For this review, use the dimensioned drawing (mm, ordinates from the lowest corner) and the shaded views. A direction names the side the tool comes from. Give positions to 0.01 mm unless a question says otherwise; leave off trailing zeros. Order: outer loops, then holes, each group sorted by start corner. A loop starts at its lowest first (then second) coordinate and runs counter-clockwise, first axis right, second up. Notation, with made-up numbers: (-24.5, 76.5) - (10.5, 76.5) arc R22 cw to (10.5, 87.5) - close; hole circle Ø5 at (26.25, -16.75). An arc over 180 degrees is marked (long way). One line per item, written item: value.
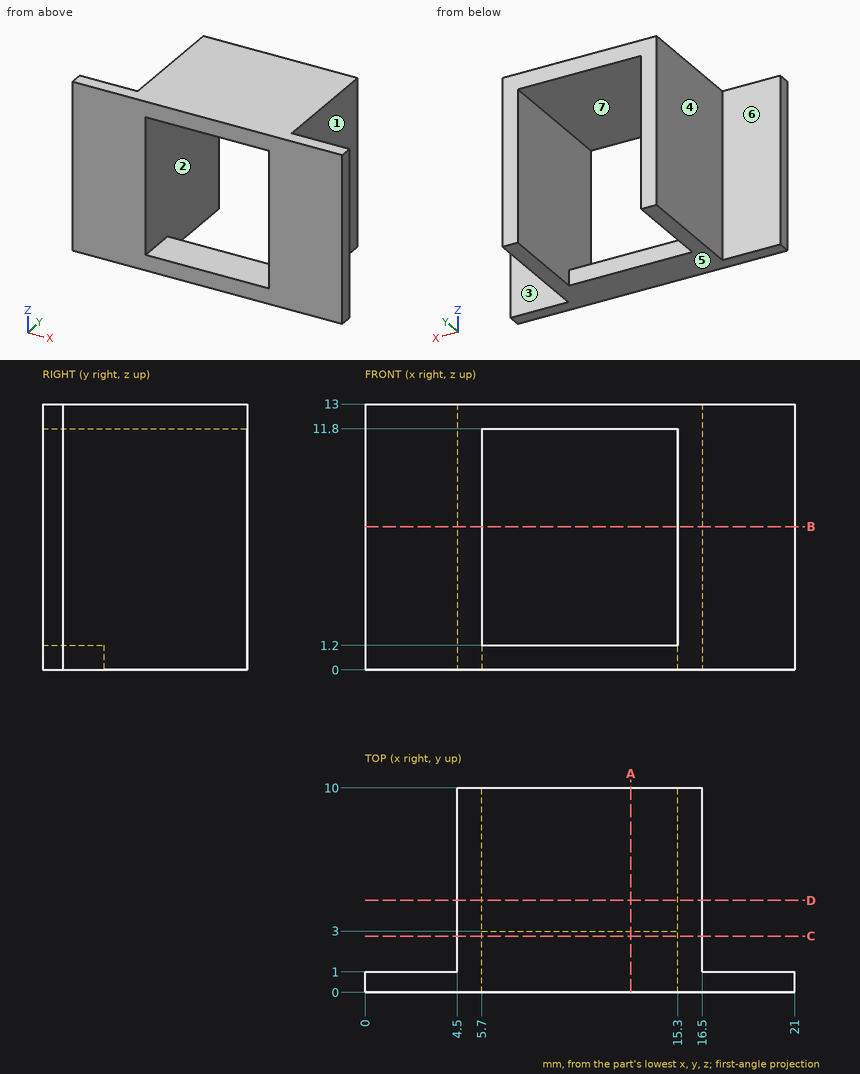
(1) Take a section at D-D (y = 4.5). Write out the cut boundary in (x, z).
Answers below:
outline: (4.5, 0) - (5.7, 0) - (5.7, 11.8) - (15.3, 11.8) - (15.3, 0) - (16.5, 0) - (16.5, 13) - (4.5, 13) - close
(2) Take a section at C-C (y = 2.75). Write out the cut boundary in (x, z).
Answers below:
outline: (4.5, 0) - (16.5, 0) - (16.5, 13) - (4.5, 13) - close; hole (5.7, 1.2) - (15.3, 1.2) - (15.3, 11.8) - (5.7, 11.8) - close
(3) Take a section at B-B (z = 7). Write out the cut boundary in (x, y).
Answers below:
outline: (0, 0) - (5.7, 0) - (5.7, 10) - (4.5, 10) - (4.5, 1) - (0, 1) - close; (15.3, 0) - (21, 0) - (21, 1) - (16.5, 1) - (16.5, 10) - (15.3, 10) - close
(4) Wall thickness on line 1 (X direction, y = 9, z = 4); line 2 (Z direction, x = 14, y = 2); line 3 (Y direction, x = 19.5, z = 10): over which ranges is each line inside the solid? List them lowest first. Write a range as from..to.
Answers below:
line 1: x = 4.5..5.7, 15.3..16.5
line 2: z = 0..1.2, 11.8..13
line 3: y = 0..1
(5) Machinability: for the marked faces 5, 6 and 7, which of the approach directions +Z, -Z, +X, -X, +Y, -Y give a long, thin tool a straight path to every point of the face, cutting with its end or side? Answer none if there is none.
Answers below:
face 5: -Z, +X, -X, +Y, -Y
face 6: +Z, -Z, -X, +Y
face 7: +Y, -Y
(6) For P1, Ø3, axis at x = 8.5, y = 6, coming from the -Z side; P2, Ø2.5, axis at y = 4.5, z = 8.5, coming from the -X side; P3, Ø4, axis at y = 8, z = 4.5, coming from the +X side, all flat-tipped, find the tip position at first contact; note any pin that passes through.
Answers below:
P1: stops at z = 11.8
P2: stops at x = 4.5
P3: stops at x = 16.5
(7) Draft analysis for pull direction X (two halves, no side actions). For the marked faces 1, 2, 3 and 4, state which applies: pulls with the +X half, pulls with the -X half, needs draft (parallel to the pull), parting line crosses it, or undercut.
Answers below:
face 1: pulls with the +X half
face 2: undercut
face 3: needs draft
face 4: pulls with the -X half
(8) Take a section at A-A (x = 13). Write out the cut boundary in (y, z), then the cut area to 3 significant figures.
Answers below:
outline: (0, 0) - (3, 0) - (3, 1.2) - (0, 1.2) - close; (0, 11.8) - (10, 11.8) - (10, 13) - (0, 13) - close
area: 15.6 mm^2
